Autodesk Inventor part; units mm, degrees
ref_plane "YZ Plane" through (0, 0, 0) normal (1, 0, 0) x (0, 1, 0)
ref_plane "XZ Plane" through (0, 0, 0) normal (0, 1, 0) x (-1, 0, 0)
ref_plane "XY Plane" through (0, 0, 0) normal (0, 0, 1) x (1, 0, 0)
sketch "Sketch1" plane through (0, 0, 0) normal (0, 1, 0) x (-1, 0, 0)
  line L0 (0, 0) -> (20, 0) construction
  circle A0 centre (20, 0) radius 1.75
  line L1 (0, 0) -> (25, 0) construction
  line L2 (25, 0) -> (25, -10) construction
  line L3 (10.2, 13.6) -> (23, 4)
  line L4 (10.2, -13.6) -> (23, -4)
  arc A1 (23, -4) -> (23, 4) centre (20, 0) ccw
  line L5 (0, 0) -> (0, -10)
  circle A2 centre (-20, 0) radius 1.75
  line L6 (-10.2, 13.6) -> (-23, 4)
  line L7 (-10.2, -13.6) -> (-23, -4)
  arc A3 (-23, 4) -> (-23, -4) centre (-20, 0) ccw
  arc A4 (10.2, 13.6) -> (-10.2, 13.6) centre (0, 0) ccw
  arc A5 (-10.2, -13.6) -> (10.2, -13.6) centre (0, 0) ccw
  dimension "d1" = 20
  dimension "d2" = 3.5
  dimension "d3" = 25
  dimension "d7" = 17
  dimension "d20" = 10
  dimension "d21" = 10
extrude "Extrusion1" add sketch "Sketch1" along normal blind 1
sketch "Sketch2" plane through (0, 1, 0) normal (0, 1, 0) x (1, 0, 0)
  circle A0 centre (0, 0) radius 15
  dimension "d11" = 30
extrude "Extrusion2" add sketch "Sketch2" along normal blind 4 and the other way blind 3
sketch "Sketch3" plane through (0, -2, 0) normal (0, -1, 0) x (1, 0, 0)
  circle A0 centre (0, 0) radius 12.7
  dimension "d15" = 25.4
extrude "Extrusion3" add sketch "Sketch3" along normal blind 15.8
properties part number "tube socket 9 pin"
The model under review builds one solid part; all positions refer to its coordinate system, in mm. A direction names the side the tool comes from. Round coordinates to 2 decimals unless told otherwise and drop trailing zeros. Order: outer loops, then holes, each group sorted by start corner. A loop starts at its lowest first (then second) coordinate and runs counter-clockwise, first axis right, second up.
Item 1: To check wall thickness, follow probe 1 along Y at (x, z) = (-18, -3.5); probe 2 along Z at (x, y) = (20, 0.75). State the ranges of each line that lie inside material, in increasing order.
Working result:
probe 1: y = 0 to 1
probe 2: z = -6.25 to -1.75, 1.75 to 6.25
Item 2: For pin 1 (8 mm diameter, centred on x = 6, y = -8, fed in from +Z); pin 2 (4 mm diameter, centred on y = 0.5, z = -9.5, fed in from +X); pin 3 (8 mm diameter, centred on x = 13, y = -3, fed in from +Z); pin 4 (3 mm diameter, centred on x = -20, z = 0, fed in from -Y), all flat-tipped, find the tip position at first contact; note any pin that passes through.
Working result:
pin 1: stops at z = 12.54
pin 2: stops at x = 18.33
pin 3: stops at z = 13.48
pin 4: passes through
Item 3: Machinability: for faces 1 (the flat face through (16.51, 0.493, -8.867)), 2 (the cylindrical face through (-14.985, -0.986, -0.66)), 3 (the flat face through (6, 1, 14)), which of the approach directions +Z, -Z, +X, -X, +Y, -Y give a long, thin tool a straight path to every point of the face, cutting with its end or side? Answer none if there is none.
Working result:
face 1: -Z, +X, +Y, -Y
face 2: -Y
face 3: +Y
Item 4: Add section A-A, the plane x = -20. State the section outline as (y, z) points, and give its area (3 significant figures).
Working result:
outline: (0, -6.25) - (1, -6.25) - (1, -1.75) - (0, -1.75) - close; (0, 1.75) - (1, 1.75) - (1, 6.25) - (0, 6.25) - close
area: 9.00 mm2
Item 5: Add section B-B, the plane z = 0. State the section outline as (x, y) points.
Working result:
outline: (-25, 0) - (-21.75, 0) - (-21.75, 1) - (-25, 1) - close; (-18.25, 0) - (-15, 0) - (-15, -2) - (-12.7, -2) - (-12.7, -17.8) - (12.7, -17.8) - (12.7, -2) - (15, -2) - (15, 0) - (18.25, 0) - (18.25, 1) - (15, 1) - (15, 5) - (-15, 5) - (-15, 1) - (-18.25, 1) - close; (21.75, 0) - (25, 0) - (25, 1) - (21.75, 1) - close
Item 6: Add section D-D, the plane z = 8. State the section outline as (x, y) points, and give its area (3 significant figures).
Working result:
outline: (-17.67, 0) - (-12.69, 0) - (-12.69, -2) - (-9.86, -2) - (-9.86, -17.8) - (9.86, -17.8) - (9.86, -2) - (12.69, -2) - (12.69, 0) - (17.67, 0) - (17.67, 1) - (12.69, 1) - (12.69, 5) - (-12.69, 5) - (-12.69, 1) - (-17.67, 1) - close
area: 499 mm2
Item 7: Add section C-C, the plane x = 0. State the section outline as (y, z) points, and give its area (3 significant figures).
Working result:
outline: (-17.8, -12.7) - (-2, -12.7) - (-2, -15) - (0, -15) - (0, -17) - (1, -17) - (1, -15) - (5, -15) - (5, 15) - (1, 15) - (1, 17) - (0, 17) - (0, 15) - (-2, 15) - (-2, 12.7) - (-17.8, 12.7) - close
area: 615 mm2
Item 8: Draft analysis for pull direction X (two halves, no side actions). For faces 4 (the cylindrical face through (25, 0.5, -0.1)), 5 (the cylindrical face through (21.75, 0.49, -0.08)), 6 (the flat face through (-16.51, 0.493, -8.867)), state which applies: released by +X, released by -X, zero draft, split by the parting line, or undercut.
Working result:
face 4: released by +X
face 5: undercut
face 6: released by -X
